Source: CAD feature listing. Evaluate the final solid. Frame: model axes, mm. Give positions to 0.01 mm unless a question says otherwise; leave off trailing zeros. Loops run counter-clockwise (first coordinate to the right, second up) from the corner with the lowest first, then second, coordinate; pieces in that order, holes last. Notation, with made-up numbers: (50, 21) - (91, 21) arc R6 ccw to (91, 27) - close; hole circle Ø6 at (-21, 30). An arc over 180 degrees is marked (long way). Write each question's results on one line, items separated by ' | '. Start each with the question number.
(1) Contact query for flat-ended pins moving along their axis: pin 1 (3 mm diameter, centred on x = 8, y = -2, fed in from -Z); pin 2 (2 mm diameter, centred on x = 14, z = 2, fed in from -Y). Output: stop coordinate, or through.
(2) Pull-direction query (X, two-part tool) for faces 1 (the flat face through (20, 0, 0)), 2 (the cylindrical face through (15.319, -1.341, -3.233)), 3 (the cylindrical face through (-1.504, -3.905, 0.867)); classes: pulls with the +X half, pulls with the -X half, needs draft (parallel to the pull), parting line crosses it, or undercut.
(3) Material intervals for line 1 along Z through (x, y) = (8, 0.25); line 2 along Z through (x, y) = (-11, -1.5), sorted ascending. Write a range as [from, to].
(4) Cut plane A-A on x = -15. Return the cut outline in (y, z), then the cut area to 3 significant figures.
from build123d import *

# Parameters (mm, degrees)
SKETCH2_R           = 4
EXTRUDE1_DEPTH      = 18.4
EXTRUDE1_DEPTH_BACK = 18.4
SKETCH3_R           = 4
EXTRUDE2_DEPTH      = 1.6
EXTRUDE2_TAPER      = 15
SKETCH4_R           = 4
EXTRUDE3_DEPTH      = 1.6
EXTRUDE3_TAPER      = 15
SKETCH5_R           = 4
SKETCH5_R_2         = 3.5
CUT_EXTRUDE1_DEPTH  = 0.8


with BuildPart() as part:
    # Sketch2 → Extrude1 (new body, two sides)
    with BuildSketch(Plane(origin=(0, 0, 0), x_dir=(0, 0, -1), z_dir=(1, 0, 0))) as extrude1_sk:
        Circle(SKETCH2_R)
    extrude(amount=EXTRUDE1_DEPTH)
    extrude(extrude1_sk.sketch, amount=-EXTRUDE1_DEPTH_BACK)

    # Sketch3 → Extrude2 (add)
    with BuildSketch(Plane(origin=(18.4, 0, 0), x_dir=(0, 0, -1), z_dir=(1, 0, 0))):
        Circle(SKETCH3_R)
    extrude(amount=EXTRUDE2_DEPTH, taper=EXTRUDE2_TAPER)

    # Sketch4 → Extrude3 (add)
    with BuildSketch(Plane.ZY.offset(18.4)):
        Circle(SKETCH4_R)
    extrude(amount=EXTRUDE3_DEPTH, taper=EXTRUDE3_TAPER)

    # Sketch5 → Cut-Extrude1 (cut)
    with BuildSketch(Plane(origin=(14.92499999, 0, 0), x_dir=(0, 0, -1), z_dir=(1, 0, 0))):
        Circle(SKETCH5_R)
        Circle(SKETCH5_R_2, mode=Mode.SUBTRACT)
    extrude(amount=CUT_EXTRUDE1_DEPTH, mode=Mode.SUBTRACT)


solid = part.part
Ans:
1) pin 1: z = -3.97 | pin 2: y = -3.87
2) face 1: pulls with the +X half | face 2: undercut | face 3: needs draft
3) line 1: [-3.99, 3.99] | line 2: [-3.71, 3.71]
4) outline: circle Ø8 at (0, 0) | area: 50.3 mm^2
